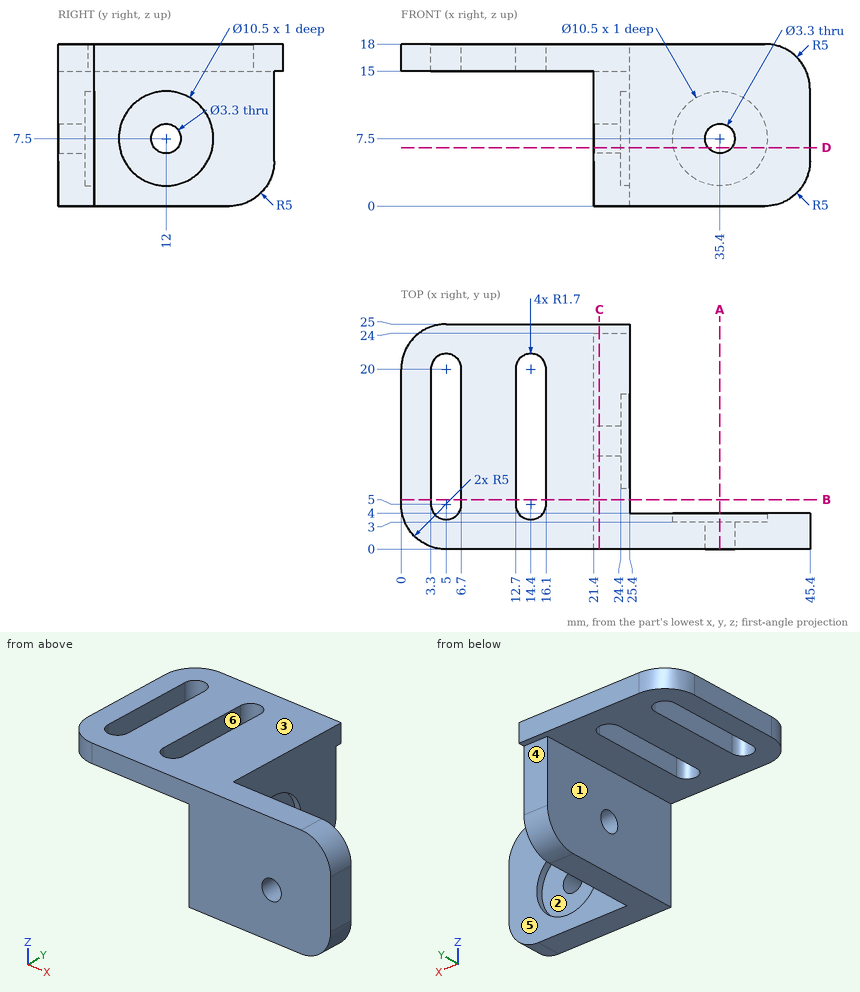
Design review of the part shown in the three views and the two pictorial views. Dimensions are in mm from the part's minimum x, y and z. A direction names the side the tool comes from. Round coordinates to 2 decimals unless told otherwise and drop trailing zeros. Write each loop counter-clockwise with the first axis right and the second up, starting at its lowest first coordinate (ties: lowest second). Pieces come first, ordered by that corner, then holes.
Item 1: Consider section C-C on x = 22. Give the boundary of the cut face in (y, z), and give its area (3 significant figures).
Item 2: Consider section D-D on z = 6.5. Give the boundary of the cut face in (x, y).
Item 3: Consider section B-B on y = 5.5. Give the boundary of the cut face in (x, z).
Item 4: Draft analysis for pull direction X (two halves, no side actions). For the marked faces 1, 2 and 3, state which applies: released by +X, released by -X, zero draft, split by the parting line, or undercut.
Item 5: Wall thickness on L1, parallel to X at y = 15.25, z = 16.75; L2, parallel to Y at x = 24.8, z = 7.5; L3, parallel to Z at x = 35.4, y = 3.55: over which ranges is each line inside the solid? List them lowest first.
Item 6: Consider section A-A on x = 35.4. Give the boundary of the cut face in (y, z).
Item 7: For the marked faces 4, 5 and 6, list the 3-axis set-ups (+Z, -Z, +X, -X, +Y, -Y) from which the entire face can be reached by the end or side of a thin tool; tool diameter is ignored.
Item 8: For pin 1 Ø0.9 at (y, z) = (14, 16.5) entering from +X; pin 2 Ø4 at (y, z) = (16, 14.5) entering from -X; pin 3 Ø3 at (x, y) = (10, 8) entering from -Z; pin 4 Ø2.5 at (y, z) = (12, 7.5) entering from -X, all flat-tipped, find the tip position at first contact; note any pin that passes through.
Check values:
1. outline: (0, 0) - (19, 0) arc R5 ccw to (24, 5) - (24, 15) - (25, 15) - (25, 18) - (0, 18) - close; hole circle Ø3.3 at (12, 7.5)
1. area: 421 mm2
2. outline: (21.4, 0) - (34.09, 0) - (34.09, 3) - (30.25, 3) - (30.25, 4) - (25.4, 4) - (25.4, 6.85) - (24.4, 6.85) - (24.4, 10.69) - (21.4, 10.69) - close; (21.4, 13.31) - (24.4, 13.31) - (24.4, 17.15) - (25.4, 17.15) - (25.4, 24) - (21.4, 24) - close; (36.71, 0) - (45.4, 0) - (45.4, 4) - (40.55, 4) - (40.55, 3) - (36.71, 3) - close
3. outline: (0, 15) - (3.3, 15) - (3.3, 18) - (0, 18) - close; (6.7, 15) - (12.7, 15) - (12.7, 18) - (6.7, 18) - close; (16.1, 15) - (21.4, 15) - (21.4, 0) - (25.4, 0) - (25.4, 18) - (16.1, 18) - close
4. face 1: released by -X
4. face 2: undercut
4. face 3: zero draft
5. L1: x = 0 to 3.3, 6.7 to 12.7, 16.1 to 25.4
5. L2: y = 0 to 6.75, 17.25 to 24
5. L3: z = 0 to 2.25, 12.75 to 18
6. outline: (0, 0) - (4, 0) - (4, 2.25) - (3, 2.25) - (3, 5.85) - (0, 5.85) - close; (0, 9.15) - (3, 9.15) - (3, 12.75) - (4, 12.75) - (4, 18) - (0, 18) - close
7. face 4: -Z, +X, -X, +Y
7. face 5: +Z, -Z, +X, +Y
7. face 6: +Z, -Z
8. pin 1: stops at x = 25.4
8. pin 2: stops at x = 0
8. pin 3: stops at z = 15
8. pin 4: passes through
